Autodesk Inventor part; units mm, degrees
ref_plane "YZ Plane" through (0, 0, 0) normal (1, 0, 0) x (0, 1, 0)
ref_plane "XZ Plane" through (0, 0, 0) normal (0, 1, 0) x (-1, 0, 0)
ref_plane "XY Plane" through (0, 0, 0) normal (0, 0, 1) x (1, 0, 0)
sketch "Boceto1" plane through (0, 0, 0) normal (0, 1, 0) x (-1, 0, 0)
  line L0 (-15, 25) -> (15, 25)
  line L1 (15, 25) -> (15, -25)
  line L2 (15, -25) -> (-15, -25)
  line L3 (-15, -25) -> (-15, 25)
  line L4 (-15, 25) -> (15, -25) construction
  line L5 (15, 25) -> (-15, -25) construction
  point P0 (0, 0)
  dimension "d0" = 30
  dimension "d1" = 50
extrude "Extrusión1" add sketch "Boceto1" along normal blind 10
fillet "Empalme1" radius 2 4 edges at (-15, 5, -25) (-15, 5, 25) (15, 5, -25) (15, 5, 25)
sketch "Boceto2" plane through (0, 10, 0) normal (0, 1, 0) x (1, 0, 0)
  circle A0 centre (-10, 0) radius 2.7
  circle A1 centre (0, 0) radius 2.7
  circle A2 centre (10, 0) radius 2.7
  dimension "d5" = 5.4
  dimension "d6" = 10
  dimension "d7" = 10
extrude "Extrusión2" cut sketch "Boceto2" against normal through all
sketch "Boceto3" plane through (0, 10, 0) normal (0, 1, 0) x (1, 0, 0)
  circle A0 centre (-9, -19) radius 2.7
  circle A1 centre (9, -19) radius 2.7
  circle A2 centre (-9, 19) radius 2.7
  circle A3 centre (9, 19) radius 2.7
  line L0 (-13, -25) -> (13, -25)
  line L1 (-15, 23) -> (-15, -23)
  line L2 (15, -23) -> (15, 23)
  line L3 (13, 25) -> (-13, 25)
  point P0 (0, 0)
  dimension "d10" = 5.4
  dimension "d11" = 6
  dimension "d12" = 6
  dimension "d13" = 6
  dimension "d14" = 6
extrude "Extrusión3" cut sketch "Boceto3" against normal through all
sketch "Boceto4" plane through (0, 10, 0) normal (0, 1, 0) x (1, 0, 0)
  circle A0 centre (-10, 0) radius 2.7
  circle A1 centre (-10, 0) radius 4.05
  circle A2 centre (0, 0) radius 2.7
  circle A3 centre (0, 0) radius 4.05
  circle A4 centre (10, 0) radius 2.7
  circle A5 centre (10, 0) radius 4.05
  line L0 (-10, 4.6765) -> (-5.95, 2.3383)
  line L1 (-5.95, 2.3383) -> (-5.95, -2.3383)
  line L2 (-5.95, -2.3383) -> (-10, -4.6765)
  line L3 (-10, -4.6765) -> (-14.05, -2.3383)
  line L4 (-14.05, -2.3383) -> (-14.05, 2.3383)
  line L5 (-14.05, 2.3383) -> (-10, 4.6765)
  line L6 (0, 4.6765) -> (4.05, 2.3383)
  line L7 (4.05, 2.3383) -> (4.05, -2.3383)
  line L8 (4.05, -2.3383) -> (0, -4.6765)
  line L9 (0, -4.6765) -> (-4.05, -2.3383)
  line L10 (-4.05, -2.3383) -> (-4.05, 2.3383)
  line L11 (-4.05, 2.3383) -> (0, 4.6765)
  line L12 (10, 4.6765) -> (14.05, 2.3383)
  line L13 (14.05, 2.3383) -> (14.05, -2.3383)
  line L14 (14.05, -2.3383) -> (10, -4.6765)
  line L15 (10, -4.6765) -> (5.95, -2.3383)
  line L16 (5.95, -2.3383) -> (5.95, 2.3383)
  line L17 (5.95, 2.3383) -> (10, 4.6765)
  dimension "d17" = 8.1
extrude "Extrusión4" cut sketch "Boceto4" against normal blind 4.5 contours A0 | A1 | L1 L2 A1 | A1 L0 L1 | A1 L5 L0 | L2 L3 A1 | A1 L4 L5 | L3 L4 A1 | A2 | A3 | L7 L8 A3 | A3 L6 L7 | A3 L11 L6 | L8 L9 A3 | A3 L10 L11 | L9 L10 A3 | A4 | A5 | L13 L14 A5 | A5 L12 L13 | A5 L17 L12 | L14 L15 A5 | A5 L16 L17 | L15 L16 A5
sketch "Boceto5" plane through (0, 10, 0) normal (0, 1, 0) x (1, 0, 0)
  circle A0 centre (-9, -19) radius 2.7
  circle A1 centre (-9, -19) radius 4.05
  line L0 (-13.6765, -18.9802) -> (-11.3211, -14.9401)
  line L1 (-11.3211, -14.9401) -> (-6.6446, -14.96)
  line L2 (-6.6446, -14.96) -> (-4.3235, -19.0198)
  line L3 (-4.3235, -19.0198) -> (-6.6789, -23.0599)
  line L4 (-6.6789, -23.0599) -> (-11.3554, -23.04)
  line L5 (-11.3554, -23.04) -> (-13.6765, -18.9802)
  point P0 (0, 0)
  dimension "d20" = 8.1
extrude "Extrusión5" cut sketch "Boceto5" against normal blind 4 contours A0 | A1 | A1 L2 L3 | A1 L1 L2 | L3 L4 A1 | A1 L0 L1 | L4 L5 A1 | A1 L5 L0
pattern_linear "Patrón rectangular1" count 2 spacing 38 along (0, 0, -1) count 2 spacing 18 along (1, 0, 0) of "Extrusión5"
properties part number "ViseA"
Design review of the part built by this model. Coordinates are the model's own, in mm. A direction names the side the tool comes from. Coordinates: 2 decimals unless noted, no trailing zeros. Loops run counter-clockwise (first coordinate to the right, second up) from the corner with the lowest first, then second, coordinate; pieces in that order, holes last.
Q1. To check wall thickness, follow line 1 (X direction, y = 9.75, z = -1.5); line 2 (X direction, y = 1.9, z = 19); line 3 (Z direction, x = 8.5, y = 8.5). State the ranges of each line that lie inside material, in increasing order.
Reported:
line 1: x = -15 to -14.05, -5.95 to -4.05, 4.05 to 5.95, 14.05 to 15
line 2: x = -15 to -11.7, -6.3 to 6.3, 11.7 to 15
line 3: z = -25 to -23.05, -14.95 to -3.81, 3.81 to 14.95, 23.05 to 25
Q2. We need section A-A on z = 0. State the section outline as (x, y) points, and give its area (3 significant figures).
Reported:
outline: (-15, 0) - (-12.7, 0) - (-12.7, 5.5) - (-14.05, 5.5) - (-14.05, 10) - (-15, 10) - close; (-7.3, 0) - (-2.7, 0) - (-2.7, 5.5) - (-4.05, 5.5) - (-4.05, 10) - (-5.95, 10) - (-5.95, 5.5) - (-7.3, 5.5) - close; (2.7, 0) - (7.3, 0) - (7.3, 5.5) - (5.95, 5.5) - (5.95, 10) - (4.05, 10) - (4.05, 5.5) - (2.7, 5.5) - close; (12.7, 0) - (15, 0) - (15, 10) - (14.05, 10) - (14.05, 5.5) - (12.7, 5.5) - close
area: 102 mm2
Q3. We need section B-B on y = 3.25. State the section outline as (x, z) points.
Reported:
outline: (-15, -23) arc R2 ccw to (-13, -25) - (13, -25) arc R2 ccw to (15, -23) - (15, 23) arc R2 ccw to (13, 25) - (-13, 25) arc R2 ccw to (-15, 23) - close; hole circle Ø5.4 at (-10, 0); hole circle Ø5.4 at (-9, -19); hole circle Ø5.4 at (-9, 19); hole circle Ø5.4 at (0, 0); hole circle Ø5.4 at (9, -19); hole circle Ø5.4 at (9, 19); hole circle Ø5.4 at (10, 0)
Q4. We need section D-D on z = 20. State the section outline as (x, y) points, and give its area (3 significant figures).
Reported:
outline: (-15, 0) - (-11.51, 0) - (-11.51, 6) - (-13.09, 6) - (-13.09, 10) - (-15, 10) - close; (-6.49, 0) - (6.49, 0) - (6.49, 6) - (4.91, 6) - (4.91, 10) - (-4.89, 10) - (-4.89, 6) - (-6.49, 6) - close; (11.51, 0) - (15, 0) - (15, 10) - (13.11, 10) - (13.11, 6) - (11.51, 6) - close
area: 174 mm2
Q5. Tool access review of faces 3 (the face through (-4.05, 8, 0)), 4 (the face through (12.575, 2.788, -0.811)): name each direction out of +Z, -Z, +X, -X, +Y, -Y from which nothing blocks a thin tool from reaching the whole face with its end or side.
Reported:
face 3: +Y
face 4: +Y, -Y
Q6. We need section C-C on x = -9. State the section outline as (y, z) points, and give its area (3 significant figures).
Reported:
outline: (0, -25) - (10, -25) - (10, -23.05) - (6, -23.05) - (6, -21.7) - (0, -21.7) - close; (0, -16.3) - (6, -16.3) - (6, -14.95) - (10, -14.95) - (10, -4.1) - (5.5, -4.1) - (5.5, -2.51) - (0, -2.51) - close; (0, 2.51) - (5.5, 2.51) - (5.5, 4.1) - (10, 4.1) - (10, 14.95) - (6, 14.95) - (6, 16.3) - (0, 16.3) - close; (0, 21.7) - (6, 21.7) - (6, 23.05) - (10, 23.05) - (10, 25) - (0, 25) - close
area: 306 mm2
Q7. For pin 1 (4 mm diameter, centred on x = 10.5, z = 1.5, fed in from +Y), flat-tipped, find the tip position at first contact; note if it passes through.
Reported:
pin 1: stops at y = 5.5
Q8. The part is to be moulded in two halves that separate along X. For faces 1 (the face through (-2, 7.78, 3.52)), 2 (the face through (14.43, 5.07, -24.4)), say which applies: +X half, -X half, draft (parallel to the pull), parting line (faces both ways), or undercut.
Reported:
face 1: undercut
face 2: +X half
